Could you check a few things on this drawing? It's one solid part, dimensions in mm from its lowest x, y, z. A direction names the side the tool comes from. Round coordinates to 2 decimals unless told otherwise and drop trailing zeros. Write each loop counter-clockwise with the first axis right and the second up, starting at its lowest first coordinate (ties: lowest second). Pieces come first, ordered by that corner, then holes. Notation, with made-up numbers: (9.25, 27.25) -> (39.25, 27.25) arc R18 cw to (39.25, 62.25) -> close; hole circle Ø2 at (49, 15.25). An arc over 180 degrees is marked (long way). Answer in a Markdown table with one row per item. Add a question column.
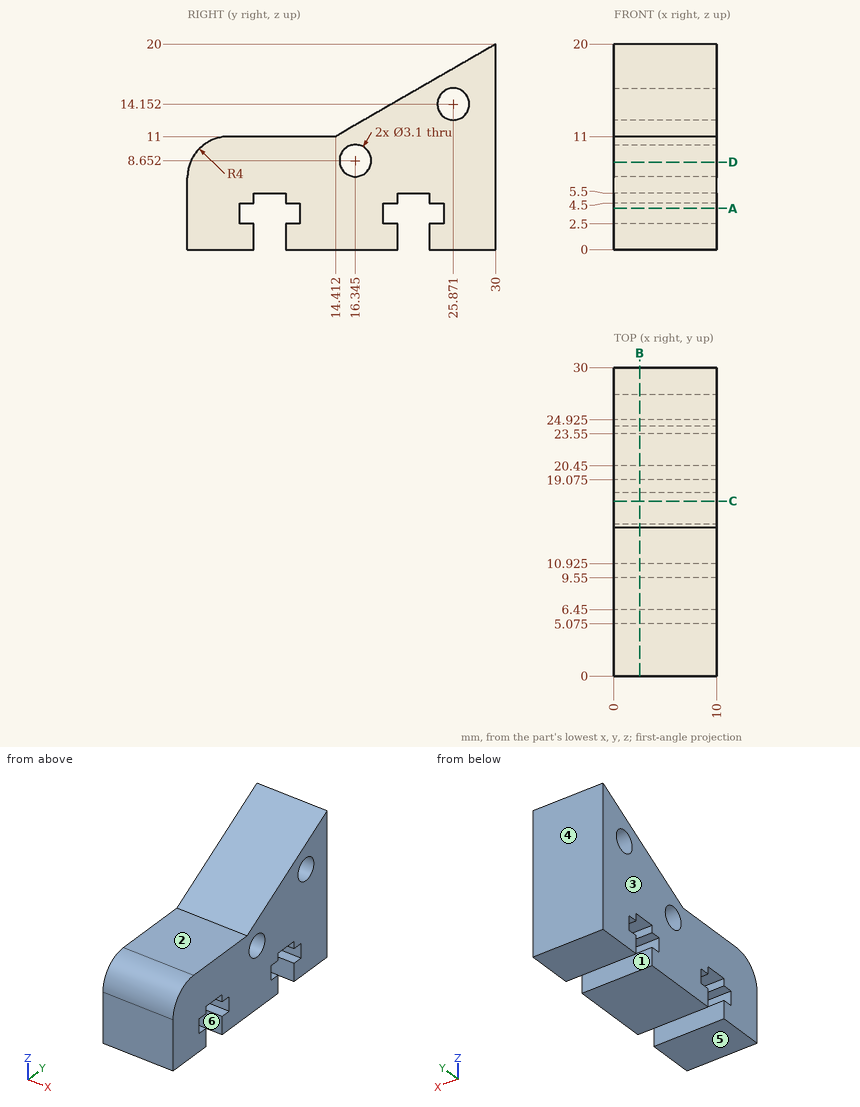
Item 1: If we mould it in two halves opening along Y, with no side actions, what happens to the marked faces 4, 5 and 6? For each: pulls with the +Y half, pulls with the -Y half, needs draft (parallel to the pull), parting line crosses it, or undercut.
Item 2: If we section it at A-A on z = 4: Please give me the cut outline in (x, y) (1 decimal), then the cut area to 3 significant figures.
Item 3: I need wall thicknesses on line 1 along Y through (x, z) = (1.75, 5); line 2 along Z through (x, y) = (5.5, 26) (1 decimal); line 3 along Y through (x, z) = (2.5, 13.5) (1 decimal). Which ranges of each line are inside material? Lowest first, please. Write a range as from..to.
Item 4: If we section it at B-B on x = 2.5: Give the number of separate pieces and of enclosed holes in the cut face.
Item 5: For P1, Ø1.5, axis at x = 5, y = 5.5, coming from the +Z side; P2, Ø4, axis at x = 2.5, z = 11.5, coming from the -Y side; P3, Ø1.6, axis at x = 3.5, y = 22, coming from the -Z side, each with a flat end and sliding along its axis, tell me the tip position at first contact or that it passes through.
Item 6: On a 3-axis mill with a long thin cutter (end or side, diameter ignored), from which of +Z, -Z, +X, -X, +Y, -Y can I reach the whole of each face in a straight line? I mean the marked faces 1, 2 and 3. Say none if no direction works.
Item 7: If we section it at C-C on y = 17: Please give me the cut outline in (x, z) (1 decimal).
Item 8: If we section it at D-D on z = 8.5: Please give me the cut outline in (x, y), then the cut area to 3 significant figures.
Results list:
| question | item | result |
|---|---|---|
| 1 | face 4 | pulls with the +Y half |
| 1 | face 5 | needs draft |
| 1 | face 6 | undercut |
| 2 | outline | (0, 0) -> (10, 0) -> (10, 5.1) -> (0, 5.1) -> close; (0, 10.9) -> (10, 10.9) -> (10, 19.1) -> (0, 19.1) -> close; (0, 24.9) -> (10, 24.9) -> (10, 30) -> (0, 30) -> close |
| 2 | area | 183 mm² |
| 3 | line 1 | 0..6.45, 9.55..20.45, 23.55..30 |
| 3 | line 2 | 0..12.6, 15.7..17.7 |
| 3 | line 3 | 18.7..24.5, 27.3..30 |
| 4 | separate pieces | 1 |
| 4 | enclosed holes | 2 |
| 5 | P1 | z = 11 |
| 5 | P2 | y = 0.88 |
| 5 | P3 | z = 5.5 |
| 6 | face 1 | -Z, +X, -X |
| 6 | face 2 | +Z, +X, -X, -Y |
| 6 | face 3 | +Z, -Z, -X, +Y, -Y |
| 7 | outline | (0, 0) -> (10, 0) -> (10, 7.2) -> (0, 7.2) -> close; (0, 10.1) -> (10, 10.1) -> (10, 12.5) -> (0, 12.5) -> close |
| 8 | outline | (0, 0.29) -> (10, 0.29) -> (10, 14.8) -> (0, 14.8) -> close; (0, 17.89) -> (10, 17.89) -> (10, 30) -> (0, 30) -> close |
| 8 | area | 266 mm² |
